Read the model definition and answer for the solid it produces. Units are mm, in the model's axes. Coordinates: 2 decimals unless noted, no trailing zeros. Order: outer loops, then holes, each group sorted by start corner. A loop starts at its lowest first (then second) coordinate and runs counter-clockwise, first axis right, second up. Notation, with made-up numbers: (-21, 2) - (9, 2) arc R31 cw to (9, 39) - close; hole circle Ø2 at (13.25, -29). An arc over 180 degrees is marked (long way). Use one line per item in the form item = value.
```python
from build123d import *

# Parameters (mm, degrees)
F3_R     = 10
F4_DEPTH = 20
F6_DEPTH = 20


with BuildPart() as f2:
    # F2: sweep along a path in F1
    with BuildLine(Plane.XY) as f2_path:
        Line((0, 0), (0, -70))
        ThreePointArc((0, -70), (43.933982822, -176.066017178), (150, -220))
        Line((150, -220), (2230, -220))
        ThreePointArc((2230, -220), (2336.066017178, -176.066017178), (2380, -70))
        Line((2380, -70), (2380, 0))
    # F0 (on Front) → F2 (sweep)
    with BuildSketch(Plane.XZ):
        with BuildLine():
            Line((0, 8.6602540378), (-5, 8.6602540378))
            ThreePointArc((-5, 8.6602540378), (-10, 0), (-5, -8.6602540378))
            Line((-5, -8.6602540378), (5, -8.6602540378))
            ThreePointArc((5, -8.6602540378), (10, 0), (5, 8.6602540378))
            Line((5, 8.6602540378), (0, 8.6602540378))
        make_face()
    sweep(path=f2_path.line)

    # F3 (on face) → F4 (join)
    with BuildSketch(Plane.XY.offset(8.6602540378)):
        with Locations((0, -70)):
            Circle(F3_R)
        with Locations((150, -220)):
            Circle(F3_R)
        with Locations((2380, -70)):
            Circle(F3_R)
        with Locations((2230, -220)):
            Circle(F3_R)
    extrude(amount=F4_DEPTH)

    # F5 (on face) → F6 (join)
    with BuildSketch(Plane.XY.offset(8.6602540378)):
        with BuildLine():
            Line((1198.6602540378, -215), (1190, -215))
            Line((1190, -215), (1190, -220))
            Line((1190, -220), (1190, -225))
            Line((1190, -225), (1198.6602540378, -225))
            ThreePointArc((1198.6602540378, -225), (1199.6592582629, -222.588190451), (1200, -220))
            ThreePointArc((1200, -220), (1199.6592582629, -217.411809549), (1198.6602540378, -215))
        make_face()
        with BuildLine():
            Line((1181.3397459622, -215), (1190, -215))
            Line((1190, -215), (1198.6602540378, -215))
            ThreePointArc((1198.6602540378, -215), (1190, -210), (1181.3397459622, -215))
        make_face()
        with BuildLine():
            Line((1190, -220), (1190, -215))
            Line((1190, -215), (1181.3397459622, -215))
            ThreePointArc((1181.3397459622, -215), (1180.3407417371, -217.411809549), (1180, -220))
            Line((1180, -220), (1190, -220))
        make_face()
        with BuildLine():
            Line((1190, -225), (1190, -220))
            Line((1190, -220), (1180, -220))
            ThreePointArc((1180, -220), (1180.3407417371, -222.588190451), (1181.3397459622, -225))
            Line((1181.3397459622, -225), (1190, -225))
        make_face()
        with BuildLine():
            Line((1198.6602540378, -225), (1190, -225))
            Line((1190, -225), (1181.3397459622, -225))
            ThreePointArc((1181.3397459622, -225), (1190, -230), (1198.6602540378, -225))
        make_face()
    extrude(amount=F6_DEPTH)


solid = f2.part
```
(1) Section B-B, the plane x = 2175 is taken. Write down the section's boundary in (y, z), then the cut area to 3 significant figures.
Answer list:
outline = (-225, -8.66) - (-215, -8.66) arc R10 ccw to (-215, 8.66) - (-225, 8.66) arc R10 ccw to start
area = 296 mm2
(2) Section A-A, the plane z = 20.5 is taken. Write down the section's boundary in (x, y), then the cut area to 3 significant figures.
Answer list:
outline = circle Ø20 at (0, -70); circle Ø20 at (150, -220); circle Ø20 at (1190, -220); circle Ø20 at (2230, -220); circle Ø20 at (2380, -70)
area = 1,570 mm2
(3) Given pin 1 Ø3 at (x, z) = (1410, 2.5) entering from +Y; pin 2 Ø3 at (y, z) = (-65.5, 15) entering from -X; pin 3 Ø5 at (x, y) = (1821.5, -218) entering from +Z; pin 4 Ø12 at (y, z) = (-180.5, 19) entering from +X, each flat-ended and moving along its own axis, determine where each tip first touches the part or whether it passes through.
Answer list:
pin_1 = -210.05
pin_2 = -9.54
pin_3 = 8.66
pin_4 = through
(4) Straight lines are drawn through the part: L1, parallel to X at y = -19, z = 2; L2, parallel to X at y = -36, z = 5; L3, parallel to Y at x = 153, z = 14. For each, find the intervals that lie inside material, in ascending order.
Answer list:
L1 = -9.8 to 9.8, 2370.2 to 2389.8
L2 = -8.66 to 8.66, 2371.34 to 2388.66
L3 = -229.54 to -210.46
